Could you check a few things on this model? Use its own coordinates, in mm. Coordinates: 2 decimals unless noted, no trailing zeros. Loops run counter-clockwise (first coordinate to the right, second up) from the corner with the lowest first, then second, coordinate; pieces in that order, holes last.
1) Imagine slicing it at A-A on y = 145. Please give me the cut outline in (x, z).
2) If I drill on line 1 along X through (y, z) = (170, 2.65); line 2 along Y through (x, z) = (-2, -1.75); line 3 along X through (y, z) = (198.85, 0) (3 decimals), over which ranges is the centre line in solid material (lowest first)?
3) Will these pins go through, and if not, where does the flat tip stop? P1, Ø2.5, axis at y = 30, z = -2.94, coming from the +X side; P2, Ø5, axis at x = 2, y = 125, coming from the -Z side; P3, Ø3.5, axis at x = 2.97, y = 15, coming from the -Z side; P4, Ø3, axis at x = 0.5, y = 98.5, coming from the -Z side.
```python
from build123d import *

# Parameters (mm, degrees)
BOSS_EXTRUDE1_DEPTH = 200
SKETCH2_W           = 12
SKETCH2_H           = 12
BOSS_EXTRUDE2_DEPTH = 5
SKETCH3_R           = 1.625
CUT_EXTRUDE1_DEPTH  = 15
CUT_EXTRUDE3_START  = -3
SKETCH6_R           = 3
CUT_EXTRUDE3_DEPTH  = 15
SKETCH7_R           = 1.5
CUT_EXTRUDE4_DEPTH  = 8
SKETCH8_R           = 1.5
CUT_EXTRUDE5_DEPTH  = 8


with BuildPart() as part:
    # Sketch1 → Boss-Extrude1 (new body)
    with BuildSketch(Plane(origin=(0, 0, 0), x_dir=(1, 0, 0), z_dir=(0, 1, 0))):
        with BuildLine():
            Line((-6, 6), (-1.5, 6))
            Line((-1.5, 6), (-1.5, 0))
            ThreePointArc((-1.5, 0), (-1.060660172, -1.060660172), (0, -1.5))
            Line((0, -1.5), (6, -1.5))
            Line((6, -1.5), (6, -6))
            Line((6, -6), (-6, -6))
            Line((-6, -6), (-6, 6))
        make_face()
    extrude(amount=BOSS_EXTRUDE1_DEPTH)

    # Sketch2 → Boss-Extrude2 (add)
    with BuildSketch(Plane(origin=(0, 200, 0), x_dir=(1, 0, 0), z_dir=(0, 1, 0))):
        Rectangle(SKETCH2_W, SKETCH2_H)
    extrude(amount=-BOSS_EXTRUDE2_DEPTH)

    # Sketch3 → Cut-Extrude1 (cut)
    with BuildSketch(Plane(origin=(0, 200, 0), x_dir=(1, 0, 0), z_dir=(0, 1, 0))):
        with Locations(Location((0, 0, 0), (0, 0, 270))):
            Circle(SKETCH3_R)
    extrude(amount=-CUT_EXTRUDE1_DEPTH, mode=Mode.SUBTRACT)

    # Sketch6 → Cut-Extrude3 (cut)
    with BuildSketch(Plane(origin=(0, 200, 0), x_dir=(1, 0, 0), z_dir=(0, 1, 0)).offset(CUT_EXTRUDE3_START)):
        with Locations(Location((0, 0, 0), (0, 0, 270))):
            Circle(SKETCH6_R)
    extrude(amount=-CUT_EXTRUDE3_DEPTH, mode=Mode.SUBTRACT)

    # Sketch7 → Cut-Extrude4 (cut)
    with BuildSketch(Plane(origin=(0, 0, 1.5), x_dir=(-1, 0, 0), z_dir=(0, 0, -1))):
        with Locations((-2.933748826, 30)):
            Circle(SKETCH7_R)
        with Locations((-2.933748826, 100)):
            Circle(SKETCH7_R)
        with Locations((-2.933748826, 170)):
            Circle(SKETCH7_R)
        with Locations((-2.966874413, 15)):
            Circle(SKETCH7_R)
    extrude(amount=-CUT_EXTRUDE4_DEPTH, mode=Mode.SUBTRACT)

    # Sketch8 → Cut-Extrude5 (cut)
    with BuildSketch(Plane(origin=(-1.5, 0, 0), x_dir=(0, 0, -1), z_dir=(1, 0, 0))):
        with Locations((2.938165571, 30)):
            Circle(SKETCH8_R)
        with Locations((2.938165571, 100)):
            Circle(SKETCH8_R)
        with Locations((2.938165571, 170)):
            Circle(SKETCH8_R)
        with Locations((2.966874413, 15)):
            Circle(SKETCH8_R)
    extrude(amount=-CUT_EXTRUDE5_DEPTH, mode=Mode.SUBTRACT)


solid = part.part
```
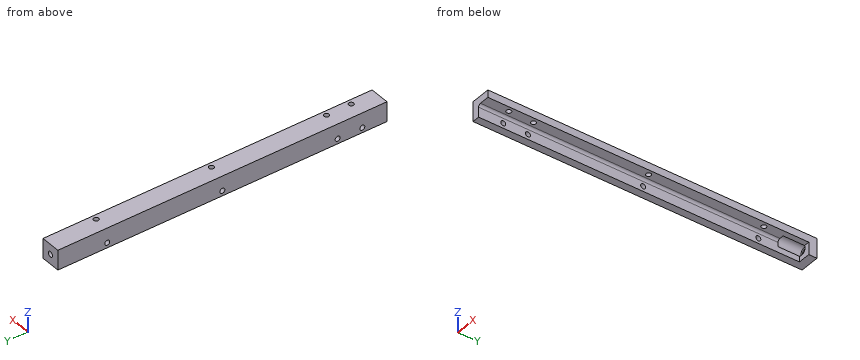
Filled in:
1. outline: (-6, -6) - (-1.5, -6) - (-1.5, 0) arc R1.5 cw to (0, 1.5) - (6, 1.5) - (6, 6) - (-6, 6) - close
2. line 1: x = -6 to 1.43, 4.43 to 6
2. line 2: y = 0 to 14.12, 15.88 to 29.08, 30.92 to 99.08, 100.92 to 169.08, 170.92 to 182, 197 to 200
2. line 3: x = -6 to -1.625, 1.625 to 6
3. P1: passes through
3. P2: stops at z = 1.41
3. P3: stops at z = 1.5
3. P4: stops at z = 1.12
